Here's how the part is built. I have some questions about the finished solid (model axes, mm). Coordinates: 2 decimals unless noted, no trailing zeros. Order: outer loops, then holes, each group sorted by start corner. A loop starts at its lowest first (then second) coordinate and runs counter-clockwise, first axis right, second up. Notation, with made-up numbers: M -3.75,83.25 L 32.25,83.25 A6 ccw 32.25,92.25 Z; hole C 13.5,28 d2. An arc over 180 degrees is marked long. One line per question, with ' | ' between items. Start each with the question number.
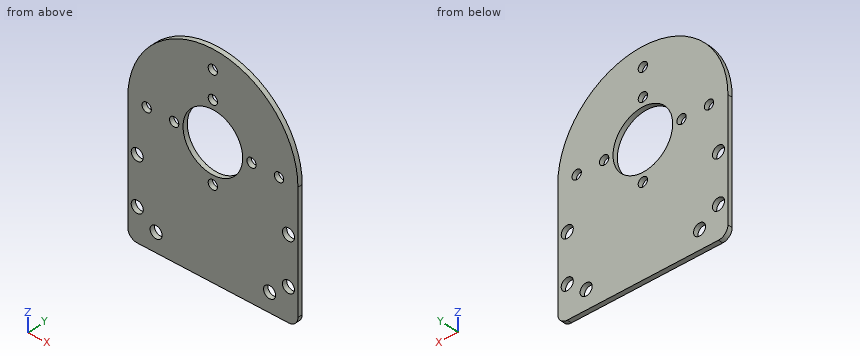
```python
from build123d import *

# Parameters (mm, degrees)
SKETCH1_R           = 10.025
SKETCH1_R_2         = 1.5625
SKETCH1_R_3         = 2.025
BOSS_EXTRUDE1_DEPTH = 1.5875


with BuildPart() as part:
    # Sketch1 → Boss-Extrude1 (new body)
    with BuildSketch(Plane(origin=(0, 0, 0), x_dir=(1, 0, 0), z_dir=(0, 1, 0))):
        with BuildLine():
            Line((-28.575, 0), (-28.575, 39.875))
            ThreePointArc((-28.575, 39.875), (-27.64506403, 42.12006403), (-25.4, 43.05))
            Line((-25.4, 43.05), (25.4, 43.05))
            ThreePointArc((25.4, 43.05), (27.64506403, 42.12006403), (28.575, 39.875))
            Line((28.575, 39.875), (28.575, 0))
            ThreePointArc((28.575, 0), (0, -28.575), (-28.575, 0))
        make_face()
        Circle(SKETCH1_R, mode=Mode.SUBTRACT)
        with Locations((0, -13)):
            Circle(SKETCH1_R_2, mode=Mode.SUBTRACT)
        with Locations((-13, 0)):
            Circle(SKETCH1_R_2, mode=Mode.SUBTRACT)
        with Locations((0, 13)):
            Circle(SKETCH1_R_2, mode=Mode.SUBTRACT)
        with Locations((13, 0)):
            Circle(SKETCH1_R_2, mode=Mode.SUBTRACT)
        with Locations((-22.225, 0)):
            Circle(SKETCH1_R_2, mode=Mode.SUBTRACT)
        with Locations((0, -22.225)):
            Circle(SKETCH1_R_2, mode=Mode.SUBTRACT)
        with Locations((22.225, 0)):
            Circle(SKETCH1_R_2, mode=Mode.SUBTRACT)
        with Locations((-25.4, 16)):
            Circle(SKETCH1_R_3, mode=Mode.SUBTRACT)
        with Locations((25.4, 16)):
            Circle(SKETCH1_R_3, mode=Mode.SUBTRACT)
        with Locations((25.4, 32)):
            Circle(SKETCH1_R_3, mode=Mode.SUBTRACT)
        with Locations((-25.4, 32)):
            Circle(SKETCH1_R_3, mode=Mode.SUBTRACT)
        with Locations((-19.05, 36.7)):
            Circle(SKETCH1_R_3, mode=Mode.SUBTRACT)
        with Locations((19.05, 36.7)):
            Circle(SKETCH1_R_3, mode=Mode.SUBTRACT)
    extrude(amount=BOSS_EXTRUDE1_DEPTH)


solid = part.part
```
1. Imagine slicing it at C-C (x = -13). List the corners of the cut face in (y, z) for me, then the cut area to 3 significant figures.
2. I need wall thicknesses on line 1 (X direction, y = 0.45, z = -16) (3 decimals); line 2 (X direction, y = 0.25, z = -17) (3 decimals); line 3 (Z direction, x = -5.5, y = 1). Which ranges of each line are inside material? Lowest first, please.
3. Imagine slicing it at A-A (z = -36.7). List the corners of the cut face in (x, y) for me (1 decimal), then the cut area to 3 significant figures.
4. Imagine slicing it at B-B (z = -13). List the corners of the cut face in (x, y) for me (1 decimal), then the cut area to 3 significant figures.
5. Imagine slicing it at D-D (y = 0.8). Count the separate pieces of the cut face and the enclosed holes in it, then the cut area to 3 significant figures.
Entries:
1) outline: M 0,-43.05 L 1.59,-43.05 L 1.59,-1.56 L 0,-1.56 Z; M 0,1.56 L 1.59,1.56 L 1.59,25.45 L 0,25.45 Z | area: 104 mm²
2) line 1: -28.575 to -27.425, -23.375 to 23.375, 27.425 to 28.575 | line 2: -28.575 to -27.161, -23.639 to 23.639, 27.161 to 28.575 | line 3: -43.05 to -8.38, 8.38 to 28.04
3) outline: M -28.6,0 L -21.1,0 L -21.1,1.6 L -28.6,1.6 Z; M -17,0 L 17,0 L 17,1.6 L -17,1.6 Z; M 21.1,0 L 28.6,0 L 28.6,1.6 L 21.1,1.6 Z | area: 77.9 mm²
4) outline: M -28.6,0 L -1.6,0 L -1.6,1.6 L -28.6,1.6 Z; M 1.6,0 L 28.6,0 L 28.6,1.6 L 1.6,1.6 Z | area: 85.8 mm²
5) separate pieces: 1 | enclosed holes: 14 | area: 3,290 mm²
